Design review of the part built by this model. Coordinates are the model's own, in mm. A direction names the side the tool comes from. Coordinates: 2 decimals unless noted, no trailing zeros. Loops run counter-clockwise (first coordinate to the right, second up) from the corner with the lowest first, then second, coordinate; pieces in that order, holes last. Notation, with made-up numbers: (80.25, 58) -> (111.25, 58) arc R27 ccw to (111.25, 74) -> close; hole circle Ø9 at (76, -23). An arc over 180 degrees is marked (long way). Answer in a Markdown table with one row per item.
```python
from build123d import *

# Parameters (mm, degrees)
SKETCH1_R           = 7.5
BOSS_EXTRUDE1_DEPTH = 22
SKETCH4_W           = 3
SKETCH4_H           = 3
CUT_EXTRUDE1_DEPTH  = 10
SKETCH5_R           = 1.5
CUT_EXTRUDE2_DEPTH  = 5
CIRPATTERN1_COUNT   = 4
BOSS_EXTRUDE2_START = -2
SKETCH6_R           = 9.5
SKETCH6_R_2         = 7.5
BOSS_EXTRUDE2_DEPTH = 2


with BuildPart() as part:
    # Sketch1 → Boss-Extrude1 (new body)
    with BuildSketch(Plane.XY):
        Circle(SKETCH1_R)
    extrude(amount=BOSS_EXTRUDE1_DEPTH)

    # Sketch4 → Cut-Extrude1 (cut)
    with BuildSketch(Plane.XY.offset(22)):
        with Locations((0, -4)):
            Rectangle(SKETCH4_W, SKETCH4_H)
    extrude(amount=-CUT_EXTRUDE1_DEPTH, mode=Mode.SUBTRACT)

    # Sketch5 → Cut-Extrude2 (cut)
    with BuildSketch(Plane(origin=(0, 0, 0), x_dir=(-1, 0, 0), z_dir=(0, 0, -1))):
        with Locations((0, 4)):
            Circle(SKETCH5_R)
    cut_extrude2 = extrude(amount=-CUT_EXTRUDE2_DEPTH, mode=Mode.SUBTRACT)

    # CirPattern1: Cut-Extrude2 ×4 about axis
    cirpattern1_axis = Axis((0, 0, 0), (0, 0, 1))
    for i in range(1, CIRPATTERN1_COUNT):
        add(cut_extrude2.rotate(cirpattern1_axis, i * 360 / CIRPATTERN1_COUNT), mode=Mode.SUBTRACT)

    # Sketch6 → Boss-Extrude2 (add)
    with BuildSketch(Plane.XY.offset(22).offset(BOSS_EXTRUDE2_START)):
        Circle(SKETCH6_R)
        Circle(SKETCH6_R_2, mode=Mode.SUBTRACT)
    extrude(amount=BOSS_EXTRUDE2_DEPTH)


solid = part.part
```
(1) To check wall thickness, follow probe 1 along Y at (x, z) = (0, 1.95); probe 2 along Z at (x, y) = (8, -5); probe 3 along X at (y, z) = (0.25, 19.5). State the ranges of each line that lie inside material, in increasing order.
Evaluation:
| item | result |
|---|---|
| probe 1 | y = -7.5 to -5.5, -2.5 to 2.5, 5.5 to 7.5 |
| probe 2 | z = 20 to 22 |
| probe 3 | x = -7.5 to 7.5 |
(2) Draft analysis for pull direction Y (two halves, no side actions). For faces 1 (the flat face through (0, 0, 22)), 2 (the cylindrical face through (4.38, -8.43, 20.99)), 3 (the cylindrical face through (5.265, 0.806, 2.465)), state which applies: pulls with the +Y half, pulls with the -Y half, needs draft (parallel to the pull), parting line crosses it, or undercut.
Evaluation:
| item | result |
|---|---|
| face 1 | needs draft |
| face 2 | parting line crosses it |
| face 3 | undercut |
(3) Take a section at D-D on y = 6.5. Give the boundary of the cut face in (x, z).
Evaluation:
| item | result |
|---|---|
| outline | (-6.93, 20) -> (-3.74, 20) -> (-3.74, 0) -> (3.74, 0) -> (3.74, 20) -> (6.93, 20) -> (6.93, 22) -> (-6.93, 22) -> close |
(4) Take a section at A-A on z = 18.75. Give the boundary of the cut face in (x, y), and give its area (3 significant figures).
Evaluation:
| item | result |
|---|---|
| outline | circle Ø15 at (0, 0); hole (-1.5, -5.5) -> (1.5, -5.5) -> (1.5, -2.5) -> (-1.5, -2.5) -> close |
| area | 168 mm² |
(5) Take a section at C-C on y = 0. Give the boundary of the cut face in (x, z).
Evaluation:
| item | result |
|---|---|
| outline | (-9.5, 20) -> (-7.5, 20) -> (-7.5, 0) -> (-5.5, 0) -> (-5.5, 5) -> (-2.5, 5) -> (-2.5, 0) -> (2.5, 0) -> (2.5, 5) -> (5.5, 5) -> (5.5, 0) -> (7.5, 0) -> (7.5, 20) -> (9.5, 20) -> (9.5, 22) -> (-9.5, 22) -> close |
(6) Tool access review of faces 4 (the flat face through (0, 4, 5)), 5 (the flat face through (0, 0, 0)), 6 (the flat face through (0, -2.5, 17)): name each direction out of +Z, -Z, +X, -X, +Y, -Y from which nothing blocks a thin tool from reaching the whole face with its end or side.
Evaluation:
| item | result |
|---|---|
| face 4 | -Z |
| face 5 | -Z, +X, -X, +Y, -Y |
| face 6 | +Z |
(7) Take a section at B-B on x = 0. Give the boundary of the cut face in (y, z).
Evaluation:
| item | result |
|---|---|
| outline | (-9.5, 20) -> (-7.5, 20) -> (-7.5, 0) -> (-5.5, 0) -> (-5.5, 5) -> (-2.5, 5) -> (-2.5, 0) -> (2.5, 0) -> (2.5, 5) -> (5.5, 5) -> (5.5, 0) -> (7.5, 0) -> (7.5, 20) -> (9.5, 20) -> (9.5, 22) -> (-2.5, 22) -> (-2.5, 12) -> (-5.5, 12) -> (-5.5, 22) -> (-9.5, 22) -> close |
(8) For pin 1 (6 mm diameter, centred on x = -1.5, z = 4.5, fed in from -Y); pin 2 (0.9 mm diameter, centred on y = -3.5, z = 19, fed in from +X); pin 3 (3.5 mm diameter, centred on x = 0, z = 14.5, fed in from +Y), all flat-tipped, find the tip position at first contact; note any pin that passes through.
Evaluation:
| item | result |
|---|---|
| pin 1 | stops at y = -7.5 |
| pin 2 | stops at x = 6.85 |
| pin 3 | stops at y = 7.5 |
